from build123d import *

# Parameters (mm, degrees)
SKETCH1_W           = 420
SKETCH1_H           = 420
SKETCH1_R           = 11
SKETCH1_W_2         = 388
SKETCH1_H_2         = 313
BOSS_EXTRUDE1_DEPTH = 3
SKETCH2_W           = 402.5
SKETCH2_H           = 332.5
SKETCH2_W_2         = 396.5
SKETCH2_H_2         = 326.5
CUT_EXTRUDE1_DEPTH  = 1
SKETCH5_R           = 2.6
SKETCH5_R_2         = 2.5
SKETCH5_R_3         = 2.4
CUT_EXTRUDE8_DEPTH  = 298


with BuildPart() as part:
    # Sketch1 → Boss-Extrude1 (new body)
    with BuildSketch(Plane(origin=(0, 0, 0), x_dir=(1, 0, 0), z_dir=(0, 1, 0))):
        Rectangle(SKETCH1_W, SKETCH1_H)
        with Locations(Location((169.75, -183.25, 0), (0, 0, 270))):
            Circle(SKETCH1_R, mode=Mode.SUBTRACT)
        Rectangle(SKETCH1_W_2, SKETCH1_H_2, mode=Mode.SUBTRACT)
    extrude(amount=BOSS_EXTRUDE1_DEPTH)

    # Sketch2 → Cut-Extrude1 (cut)
    with BuildSketch(Plane.XZ):
        Rectangle(SKETCH2_W, SKETCH2_H)
        Rectangle(SKETCH2_W_2, SKETCH2_H_2, mode=Mode.SUBTRACT)
    extrude(amount=-CUT_EXTRUDE1_DEPTH, mode=Mode.SUBTRACT)

    # Sketch5 → Cut-Extrude8 (cut, through all)
    with BuildSketch(Plane(origin=(0, 3, 0), x_dir=(1, 0, 0), z_dir=(0, 1, 0))):
        with Locations(Location((-205.5, 14.63, 0), (0, 0, 270))):
            Circle(SKETCH5_R)
        with Locations(Location((-198.5, 14.63, 0), (0, 0, 270))):
            Circle(SKETCH5_R)
        with Locations(Location((198.5, 14.63, 0), (0, 0, 270))):
            Circle(SKETCH5_R)
        with Locations(Location((205.5, 14.63, 0), (0, 0, 270))):
            Circle(SKETCH5_R)
        with Locations(Location((-11, 160.5, 0), (0, 0, 270))):
            Circle(SKETCH5_R_2)
        with Locations(Location((11, 160.5, 0), (0, 0, 270))):
            Circle(SKETCH5_R_2)
        with Locations(Location((-11, -174.5, 0), (0, 0, 270))):
            Circle(SKETCH5_R_3)
        with Locations(Location((11, -174.5, 0), (0, 0, 270))):
            Circle(SKETCH5_R_3)
    extrude(amount=-CUT_EXTRUDE8_DEPTH, mode=Mode.SUBTRACT)


solid = part.part
The listing builds one solid part. Answer for the finished solid, in the listing's coordinates (mm). Round coordinates to 2 decimals unless told otherwise and drop trailing zeros. Write each loop counter-clockwise with the first axis right and the second up, starting at its lowest first coordinate (ties: lowest second). Pieces come first, ordered by that corner, then holes. Notation, with made-up numbers: M -40,53.25 L 1,53.25 A14 cw 1,59.25 Z; hole C 0.5,11.25 d2. An arc over 180 degrees is marked long. Write each question's results on one line, items separated by ' | '. Start each with the question number.
(1) The part is cut by section D-D, the plane x = 169.75. Write down the section's boundary in (y, z).
(2) The part is cut by section C-C, the plane y = 2.05. Give the number of separate pieces and of enclosed holes in the cut face, and give its area (3 significant figures).
(3) The part is cut by section A-A, the plane x = -1.5. Write down the section's boundary in (y, z), and give its area (3 significant figures).
(4) The part is cut by section B-B, the plane z = -75. Write down the section's boundary in (x, y).
(5) Find the intervals of material crossed by line 1 (Z direction, x = 0, y = 0.25); line 2 (X direction, y = 0.5, z = 106); line 3 (X direction, y = 1.95, z = -14.63), in increasing order.
(6) Determine the mould class of faces 1 (the cylindrical face through (177.18, 1.48, 175.14)), 2 (the flat face through (-32, 0, 170)) for opening direction X: +X half, -X half, draft (parallel to the pull), parting line (faces both ways), or undercut.
Worked answers:
1) outline: M 0,-210 L 3,-210 L 3,-156.5 L 0,-156.5 L 0,-163.25 L 1,-163.25 L 1,-166.25 L 0,-166.25 Z; M 0,156.5 L 3,156.5 L 3,172.25 L 0,172.25 L 0,166.25 L 1,166.25 L 1,163.25 L 0,163.25 Z; M 0,194.25 L 3,194.25 L 3,210 L 0,210 Z
2) separate pieces: 1 | enclosed holes: 10 | area: 54,400 mm²
3) outline: M 0,-210 L 3,-210 L 3,-156.5 L 0,-156.5 L 0,-163.25 L 1,-163.25 L 1,-166.25 L 0,-166.25 Z; M 0,156.5 L 3,156.5 L 3,210 L 0,210 L 0,166.25 L 1,166.25 L 1,163.25 L 0,163.25 Z | area: 315 mm²
4) outline: M -210,0 L -201.25,0 L -201.25,1 L -198.25,1 L -198.25,0 L -194,0 L -194,3 L -210,3 Z; M 194,0 L 198.25,0 L 198.25,1 L 201.25,1 L 201.25,0 L 210,0 L 210,3 L 194,3 Z
5) line 1: z = -210 to -166.25, -163.25 to -156.5, 156.5 to 163.25, 166.25 to 210 | line 2: x = -210 to -201.25, -198.25 to -194, 194 to 198.25, 201.25 to 210 | line 3: x = -210 to -208.1, -202.9 to -201.1, -195.9 to -194, 194 to 195.9, 201.1 to 202.9, 208.1 to 210
6) face 1: undercut | face 2: draft
